Autodesk Inventor part; units mm, degrees
ref_plane "YZ Plane" through (0, 0, 0) normal (1, 0, 0) x (0, 1, 0)
ref_plane "XZ Plane" through (0, 0, 0) normal (0, 1, 0) x (-1, 0, 0)
ref_plane "XY Plane" through (0, 0, 0) normal (0, 0, 1) x (1, 0, 0)
sketch "Sketch1" plane through (0, 0, 0) normal (0, 1, 0) x (-1, 0, 0)
  circle A0 centre (0, 0) radius 23
  circle A1 centre (0, 0) radius 20
  dimension "d0" = 3
  dimension "d1" = 40
extrude "Extrusion1" add sketch "Sketch1" along normal blind 90
sketch "Sketch2" plane through (0, 0, 0) normal (0, 0, 1) x (1, 0, 0)
  line L0 (-23, 100) -> (0, 100)
  line L1 (0, 100) -> (0, 40)
  line L2 (0, 40) -> (-23, 40)
  line L3 (-23, 40) -> (-23, 100)
  line L4 (23, 90) -> (-23, 90)
  line L5 (-23, 0) -> (23, 0)
  point P0 (0, 0)
  dimension "d4" = 60
  dimension "d34" = 40
extrude "Extrusion2" cut sketch "Sketch2" along normal mid plane 20
fillet "Fillet1" radius 5 2 edges at (-19.0164, 40, 10) (-19.0164, 40, -10)
sketch "Sketch3" plane through (0, 0, 0) normal (1, 0, 0) x (0, 1, 0)
  line L0 (-21, 0) -> (126, 0)
  line L1 (105, -5) -> (105, 5)
  line L2 (90, 20) -> (90, -20)
  line L3 (0, 23) -> (0, -23)
  point P0 (0, 0)
  point P1 (50, 0)
  point P2 (20, 0)
  dimension "d9" = 30
  dimension "d31" = 20
hole "Hole1" at (0, 50, 0) at (0, 20, 0) direction (1, 0, 0) diameter 4.5 end through all
sketch "Sketch4" plane through (0, 90, 0) normal (0, 1, 0) x (0, 0, -1)
  arc A0 (-10, 17.3205) -> (10, 17.3205) centre (0, 0) ccw
  arc A1 (-10, 20.7123) -> (10, 20.7123) centre (0, 0) ccw
  circle A2 centre (0, 0) radius 20
  line L0 (10, 20.7123) -> (10, 17.3205)
  line L1 (-10, 17.3205) -> (-10, 20.7123)
  line L2 (-19.3649, -5) -> (-23, -5)
  line L3 (-23, -5) -> (-23, 5)
  line L4 (-23, 5) -> (-19.3649, 5)
  line L5 (-19.3649, 5) -> (-19.3649, -5)
  dimension "d32" = 10
  dimension "d33" = 5
extrude "Extrusion3" cut sketch "Sketch4" against normal blind 15 contours L5 A0 | A0 L2 A1 L4 | A1 L3 L4 | L2 L3 A1
fillet "Fillet2" radius 5 2 edges at (5, 75, 20.9074) (-5, 75, 20.9074)
sketch "Sketch5" plane through (0, 0, 0) normal (0, 0, 1) x (1, 0, 0)
  line L0 (23, 90) -> (3, 90)
  line L1 (3, 90) -> (3, 60)
  line L2 (3, 60) -> (23, 60)
  line L3 (23, 60) -> (23, 90)
  line L4 (23, 0) -> (23, 90)
  line L5 (23, 90) -> (-20.7123, 90)
  point P0 (0, 0)
  point P1 (22.4499, 110)
  point P2 (22.4499, 110)
  dimension "d25" = 0
  dimension "d26" = 20
  dimension "d27" = 30
extrude "Extrusion4" [suppressed]
fillet "Fillet3" [suppressed]
properties part number "Pancake_PVC Pipe 2" material "PVC-Piping"
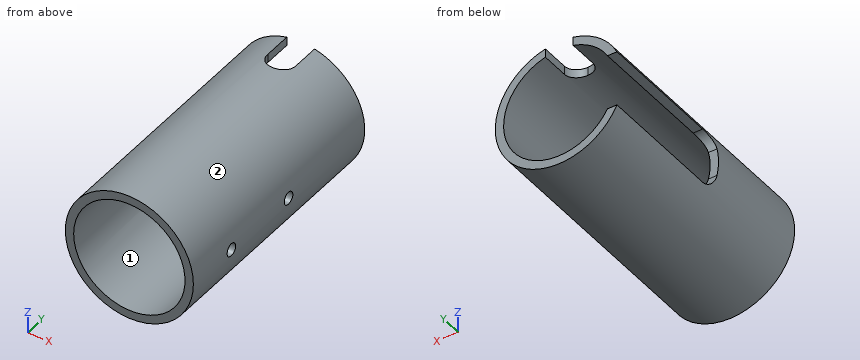
CAD build for the part. Positions are in the model's coordinates, mm. Face numbers are marked on the shaded views. Round coordinates to 2 decimals unless told otherwise and drop trailing zeros. Order: outer loops, then holes, each group sorted by start corner. A loop starts at its lowest first (then second) coordinate and runs counter-clockwise, first axis right, second up.
Item 1: Saw through at D-D on y = 20. Write the cut outline in (x, z), then the cut area to 3 significant figures.
Item 2: Saw through at B-B on x = -1. Write the cut outline in (y, z).
Item 3: Saw through at A-A on z = 0. Write the cut outline in (x, y), then the cut area to 3 significant figures.
Item 4: Pin check, flat tips, straight feed: pin 1 (1.1 mm diameter, centred on x = -21.5, z = 0, fed in from +Y); pin 2 (1 mm diameter, centred on y = 74, z = -1.5, fed in from -X); pin 3 (1 mm diameter, centred on x = -19, y = 60, fed in from -Z). Stop position of each tip, or through.
Item 5: Mould opens along Z. For the marked faces 1 and 2 say: pulls with the +Z half, pulls with the -Z half, needs draft (parallel to the pull), parting line crosses it, or undercut.
Item 6: Saw through at C-C on z = -8. Write the cut outline in (x, y).
Item 7: Probe line 1 along Z through (x, y) = (0, 39); line 2 along Z through (x, y) = (-20.5, 65); line 3 along X through (y, z) = (21.5, 0). List the from-to ranges inside material, lowest first.
Reported:
1. outline: (19.87, -2.25) arc R20 cw (long way) to (19.87, 2.25) - (22.89, 2.25) arc R23 ccw (long way) to (22.89, -2.25) - close
1. area: 392 mm2
2. outline: (0, -22.98) - (90, -22.98) - (90, -19.97) - (0, -19.97) - close; (0, 19.97) - (75.1, 19.97) - (75.1, 22.98) - (0, 22.98) - close
3. outline: (-23, 0) - (-20, 0) - (-20, 40) - (-23, 40) - close; (20, 0) - (23, 0) - (23, 17.75) - (20, 17.75) - close; (20, 22.25) - (23, 22.25) - (23, 47.75) - (20, 47.75) - close; (20, 52.25) - (23, 52.25) - (23, 90) - (20, 90) - close
3. area: 363 mm2
4. pin 1: stops at y = 40
4. pin 2: stops at x = 19.9
4. pin 3: stops at z = -13.67
5. face 1: undercut
5. face 2: parting line crosses it
6. outline: (-21.56, 0) - (-18.33, 0) - (-18.33, 41) - (-21.56, 41) - close; (18.33, 0) - (21.56, 0) - (21.56, 90) - (18.33, 90) - close
7. line 1: z = -23 to -20, 20 to 23
7. line 2: z = -10.43 to -10, 10 to 10.43
7. line 3: x = -23 to -20
